Verification items for the finished model (mm, model axes). Face numbers are marked on the shaded views. Coordinates: 2 decimals unless noted, no trailing zeros. Order: outer loops, then holes, each group sorted by start corner. A loop starts at its lowest first (then second) coordinate and runs counter-clockwise, first axis right, second up. Notation, with made-up numbers: (57, 5) -> (91, 5) arc R24 ccw to (91, 19) -> close; hole circle Ø1 at (-21, 5.5). An arc over 180 degrees is marked (long way). Write item = value, one per line. Start each with the question number.
1. Cross-section at C-C on z = 12.5. Record the cut outline in (x, y), plus the area to 3 significant figures.
2. Thickness scan on line 1 along Z through (x, y) = (32.5, 28); line 2 along Z through (x, y) = (70, 12.5); line 3 along X through (y, z) = (7, 2). Record the ranges inside material, lowest first. Write a range as from..to.
3. Release check for a two-part mould opening along Y. For the marked faces 1 and 2 record: +Y half, -Y half, draft (parallel to the pull), parting line (faces both ways), or undercut.
4. Cross-section at D-D on y = 5.5. Record the cut outline in (x, z).
5. Cross-section at B-B on x = 104.5. Record the cut outline in (y, z), plus the area to 3 significant figures.
6. Cross-section at A-A on y = 1. Record the cut outline in (x, z).
7. Go/stop test with flat-tipped pins: P1, Ø4, axis at x = 103, z = 1, coming from the +Y side; P2, Ø3.5, axis at x = 103.77, y = 0, coming from the +Z side; P3, Ø6, axis at x = 81.5, z = 3, coming from the +Y side; P4, Ø1.8, axis at x = 63.5, z = 1, coming from the +Y side. Record where each tip stops, or that it passes through.
from build123d import *

# Parameters (mm, degrees)
SKETCH_1_W          = 100.539230484
SKETCH_1_H          = 40
SKETCH_1_W_2        = 17
SKETCH_1_H_2        = 7
EXTRUDE_1_DEPTH     = 2
SKETCH_2_W          = 100.539230484
SKETCH_2_H          = 40
SKETCH_2_R          = 2.25
EXTRUDE_2_DEPTH     = 1.5
SKETCH_3_W          = 184.808915215
SKETCH_3_H          = 94.825170589
CUT_EXTRUDE_1_DEPTH = 31.5
SKETCH_4_R          = 3.5
EXTRUDE_3_DEPTH     = 10


with BuildPart() as part:
    # Эскиз1 → Бобышка-Вытянуть1 (new body)
    with BuildSketch(Plane.XY):
        with Locations((62.5, 12.5)):
            Rectangle(SKETCH_1_W, SKETCH_1_H)
        with Locations((24.230384758, 25)):
            Rectangle(SKETCH_1_W_2, SKETCH_1_H_2, mode=Mode.SUBTRACT)
        with Locations((100.769615242, 0)):
            Rectangle(SKETCH_1_W_2, SKETCH_1_H_2, mode=Mode.SUBTRACT)
    extrude(amount=EXTRUDE_1_DEPTH)

    # Эскиз2 → Бобышка-Вытянуть2 (add)
    with BuildSketch(Plane.XY.offset(2)):
        with Locations((62.5, 12.5)):
            Rectangle(SKETCH_2_W, SKETCH_2_H)
        with Locations((21.230384758, 25)):
            Circle(SKETCH_2_R, mode=Mode.SUBTRACT)
        with Locations((103.769615242, 0)):
            Circle(SKETCH_2_R, mode=Mode.SUBTRACT)
    extrude(amount=EXTRUDE_2_DEPTH)

    # Эскиз3 → Вырез-Вытянуть1 (cut)
    with BuildSketch(Plane.XY.offset(3.5)):
        with Locations((81.231416835, 7.831688581)):
            Rectangle(SKETCH_3_W, SKETCH_3_H)
        Polygon((12.230384758, 32.5), (42.230384758, 32.5), (54.020384758, 20.71), (75.769615242, 20.71), (88.979615242, 7.5), (112.769615242, 7.5), (112.769615242, -7.5), (82.769615242, -7.5), (66.982818678, 8.286796564), (45.230384758, 8.286796564), (36.017181322, 17.5), (12.230384758, 17.5), align=None, mode=Mode.SUBTRACT)
    extrude(amount=-CUT_EXTRUDE_1_DEPTH, mode=Mode.SUBTRACT)

    # Эскиз4 → Бобышка-Вытянуть3 (add)
    with BuildSketch(Plane.XY.offset(3.5)):
        with Locations((32.230384758, 28.5)):
            Circle(SKETCH_4_R)
    extrude(amount=EXTRUDE_3_DEPTH)


solid = part.part
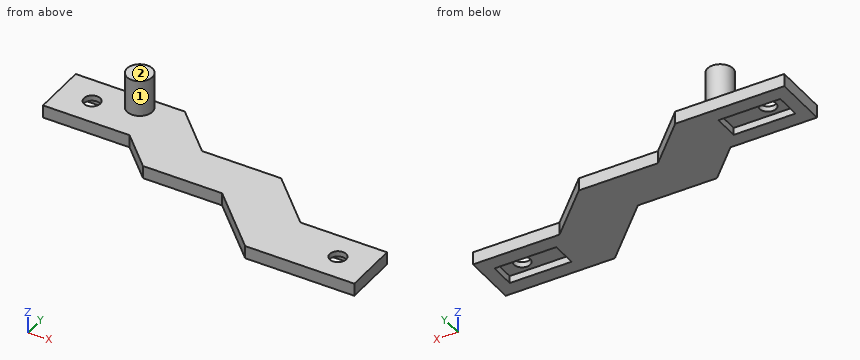
Worked out:
q1.outline = circle Ø7 at (32.23, 28.5)
q1.area = 38.5 mm²
q2.line_1 = 2..13.5
q2.line_2 = 0..3.5
q2.line_3 = 68.27..112.77
q3.face_1 = parting line
q3.face_2 = draft
q4.outline = (69.77, 0) -> (112.77, 0) -> (112.77, 3.5) -> (69.77, 3.5) -> close
q5.outline = (-7.5, 0) -> (-3.5, 0) -> (-3.5, 2) -> (-2.13, 2) -> (-2.13, 3.5) -> (-7.5, 3.5) -> close; (2.13, 2) -> (3.5, 2) -> (3.5, 0) -> (7.5, 0) -> (7.5, 3.5) -> (2.13, 3.5) -> close
q5.area = 32.1 mm²
q6.outline = (74.27, 0) -> (92.27, 0) -> (92.27, 2) -> (101.75, 2) -> (101.75, 3.5) -> (74.27, 3.5) -> close; (105.79, 2) -> (109.27, 2) -> (109.27, 0) -> (112.77, 0) -> (112.77, 3.5) -> (105.79, 3.5) -> close
q7.P1 = 7.5
q7.P2 = through
q7.P3 = 17.98
q7.P4 = 20.71
